Source: three-view drawing plus pictorial views. Frame: mm from the lowest corner of the part. Round coordinates to 2 decimals unless told otherwise and drop trailing zeros. Order: outer loops, then holes, each group sorted by start corner. A loop starts at its lowest first (then second) coordinate and runs counter-clockwise, first axis right, second up. Notation, with made-up numbers: M 88.25,70 L 128.25,70 A20 cw 128.25,83 Z; hole C 75,22.25 d10. An arc over 180 degrees is marked long. Return JSON: item names as keys, results as strings. Group by question number.
Q1. Cut plane C-C on z = 1.3. Output: boundary loops of the cut face in (x, y).
Q2. Ray query, probe 1 along Y at (x, z) = (4, 0.55); probe 2 along Y at (x, z) = (62, 2.3); probe 3 along Y at (x, z) = (38, 1.95). Return the intervals inside material, ascending.
Q3. Cut plane D-D on y = 22.5. Output: boundary loops of the cut face in (x, z), and give its area (3 significant figures).
Q4. Contact query for flat-ended pins moving along their axis: pin 1 (3.5 mm diameter, centred on x = 62, y = 42, fed in from +Z); pin 2 (2.5 mm diameter, centred on x = 4, y = 42, fed in from -Z). Output: stop coordinate, or through.
Q5. Cut plane B-B on x = 62. Output: boundary loops of the cut face in (y, z).
Q6. Cut plane A-A on y = 42. Output: boundary loops of the cut face in (x, z), and give its area (3 significant figures).
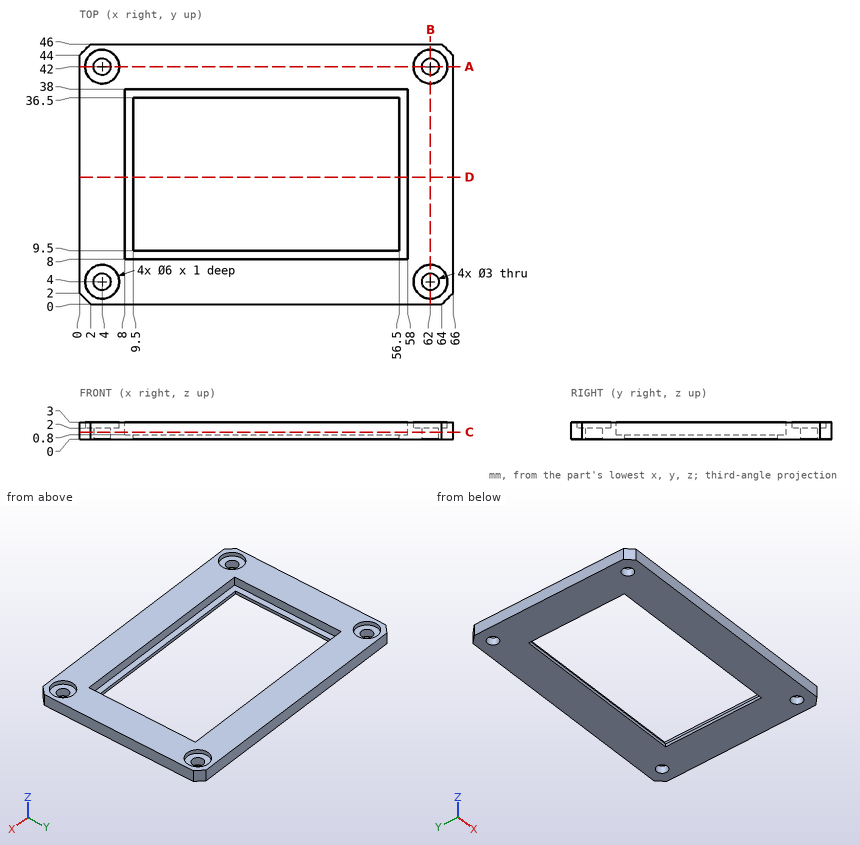
Result sheet:
{
 "1": {"outline": "M 0,2 L 2,0 L 64,0 L 66,2 L 66,44 L 64,46 L 2,46 L 0,44 Z; hole C 4,4 d3; hole C 4,42 d3; hole M 8,8 L 58,8 L 58,38 L 8,38 Z; hole C 62,4 d3; hole C 62,42 d3"},
 "2": {"probe 1": "y = 0 to 2.5, 5.5 to 40.5, 43.5 to 46", "probe 2": "y = 0 to 1, 7 to 39, 45 to 46", "probe 3": "y = 0 to 8, 38 to 46"},
 "3": {"outline": "M 0,0 L 9.5,0 L 9.5,0.8 L 8,0.8 L 8,3 L 0,3 Z; M 56.5,0 L 66,0 L 66,3 L 58,3 L 58,0.8 L 56.5,0.8 Z", "area": "50.4 mm²"},
 "4": {"pin 1": "stops at z = 2", "pin 2": "passes through"},
 "5": {"outline": "M 0,0 L 2.5,0 L 2.5,2 L 1,2 L 1,3 L 0,3 Z; M 5.5,0 L 40.5,0 L 40.5,2 L 39,2 L 39,3 L 7,3 L 7,2 L 5.5,2 Z; M 43.5,0 L 46,0 L 46,3 L 45,3 L 45,2 L 43.5,2 Z"},
 "6": {"outline": "M 0,0 L 2.5,0 L 2.5,2 L 1,2 L 1,3 L 0,3 Z; M 5.5,0 L 60.5,0 L 60.5,2 L 59,2 L 59,3 L 7,3 L 7,2 L 5.5,2 Z; M 63.5,0 L 66,0 L 66,3 L 65,3 L 65,2 L 63.5,2 Z", "area": "174 mm²"}
}
